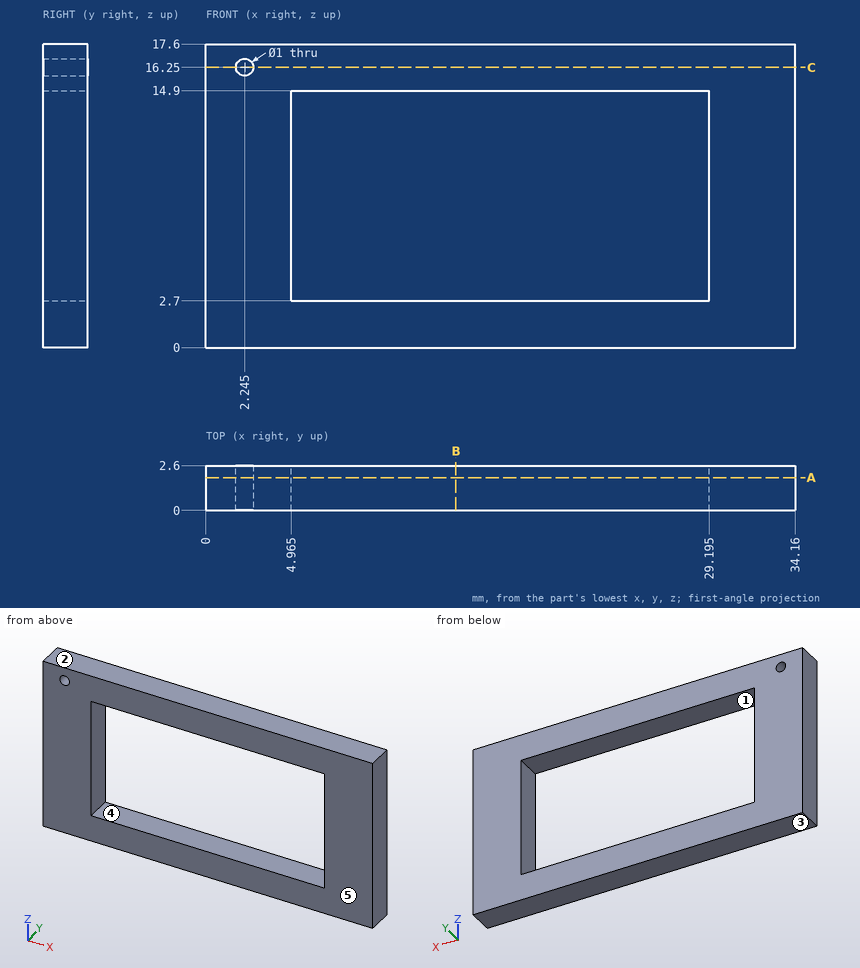
Could you check a few things on this drawing? It's one solid part, dimensions in mm from its lowest x, y, z. A direction names the side the tool comes from. Round coordinates to 2 decimals unless told otherwise and drop trailing zeros. Order: outer loops, then holes, each group sorted by start corner. A loop starts at its lowest first (then second) coordinate and runs counter-clockwise, first axis right, second up.
Q1. Please list where these lines run through material, in increasing order: probe 1 along X at (y, z) = (0.35, 4) (3 decimals); probe 2 along X at (y, z) = (0.65, 16.25) (3 decimals); probe 3 along Z at (x, y) = (8, 2.1).
Geometry says:
probe 1: x = 0 to 4.965, 29.195 to 34.16
probe 2: x = 0 to 1.745, 2.745 to 34.16
probe 3: z = 0 to 2.7, 14.9 to 17.6
Q2. Imagine slicing it at C-C, the plane z = 16.25. List the corners of the cut face in (x, y) for me (3 decimals).
Geometry says:
outline: (0, 0) - (1.745, 0) - (1.745, 2.6) - (0, 2.6) - close; (2.745, 0) - (34.16, 0) - (34.16, 2.6) - (2.745, 2.6) - close
Q3. Which directions (+Z, -Z, +X, -X, +Y, -Y) give clear straight access to the entire face, cutting with the end or side of a thin tool? Please do the marked faces 1 and 2.
Geometry says:
face 1: +Y, -Y
face 2: +Z, +X, -X, +Y, -Y
Q4. Imagine slicing it at B-B, the plane x = 14.5. List the corners of the cut face in (y, z) for me.
Geometry says:
outline: (0, 0) - (2.6, 0) - (2.6, 2.7) - (0, 2.7) - close; (0, 14.9) - (2.6, 14.9) - (2.6, 17.6) - (0, 17.6) - close
Q5. Thinking about a two-plate mould opening in Z: for the marked faces 3, 4 and 5, which applies, released by +Z, released by -Z, zero draft, split by the parting line, or undercut?
Geometry says:
face 3: released by -Z
face 4: undercut
face 5: zero draft
Q6. Imagine slicing it at A-A, the plane y = 1.9. List the corners of the cut face in (x, z) for me (3 decimals).
Geometry says:
outline: (0, 0) - (34.16, 0) - (34.16, 17.6) - (0, 17.6) - close; hole circle Ø1 at (2.245, 16.25); hole (4.965, 2.7) - (29.195, 2.7) - (29.195, 14.9) - (4.965, 14.9) - close
